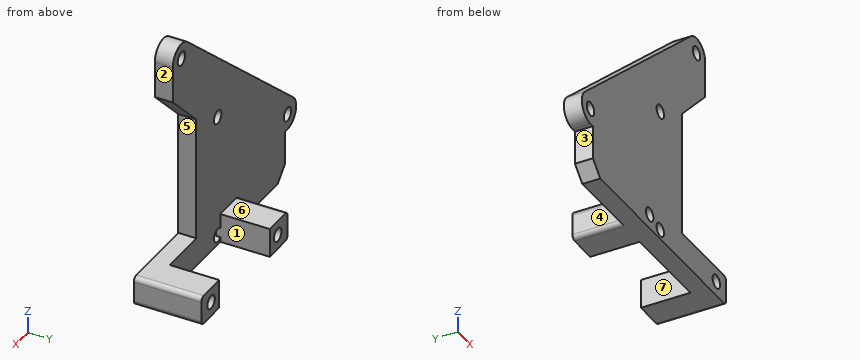
from build123d import *

# Parameters (mm, degrees)
CYLINDER035_R          = 1.5
CYLINDER035_DEPTH      = 30
CYLINDER035_ROLL_ANGLE = -90
CYLINDER034_R          = 1.5
CYLINDER034_DEPTH      = 30
CYLINDER034_ROLL_ANGLE = -90
BOX033_W               = 7.25
BOX033_H               = 12
BOX033_DEPTH           = 6.5
BOX032_W               = 7.25
BOX032_H               = 12
BOX032_DEPTH           = 6.5
SKETCH019_R            = 1.5
PAD017_DEPTH           = 4
FILLET027_R            = 1
CHAMFER008_SIZE        = 3


with BuildPart() as cylinder035:
    # Cylinder035 → Cylinder035 (new body)
    with BuildSketch(Plane.XY):
        Circle(CYLINDER035_R)
    extrude(amount=CYLINDER035_DEPTH)


with BuildPart() as cylinder035_1:
    # Cylinder035 roll: moved
    add(cylinder035.part.rotate(Axis((0, 0, 0), (1, 0, 0)), CYLINDER035_ROLL_ANGLE))


with BuildPart() as cylinder035_2:
    # Cylinder035 placement: moved
    add(cylinder035_1.part.moved(Location((-25, 27, -34.75))))


with BuildPart() as fusion031:
    # Cylinder034 → Cylinder034 (new body)
    with BuildSketch(Plane.XY):
        Circle(CYLINDER034_R)
    extrude(amount=CYLINDER034_DEPTH)


with BuildPart() as fusion031_1:
    # Cylinder034 roll: moved
    add(fusion031.part.rotate(Axis((0, 0, 0), (1, 0, 0)), CYLINDER034_ROLL_ANGLE))


with BuildPart() as fusion031_2:
    # Cylinder034 placement: moved
    add(fusion031_1.part.moved(Location((2, 27, -34.75))))

    # Fusion031: union Cylinder035
    add(cylinder035_2.part)


with BuildPart() as cube033:
    # Box033 → Box033 (new body)
    with BuildSketch(Plane(origin=(-29, 33, -38), x_dir=(1, 0, 0), z_dir=(0, 0, 1))):
        with Locations((3.625, 6)):
            Rectangle(BOX033_W, BOX033_H)
    extrude(amount=BOX033_DEPTH)


with BuildPart() as cube032:
    # Box032 → Box032 (new body)
    with BuildSketch(Plane(origin=(-1.25, 33, -38), x_dir=(1, 0, 0), z_dir=(0, 0, 1))):
        with Locations((3.625, 6)):
            Rectangle(BOX032_W, BOX032_H)
    extrude(amount=BOX032_DEPTH)


with BuildPart() as chamfer008:
    # Sketch019 → Pad017 (new body)
    with BuildSketch(Plane(origin=(0, 30, 0), x_dir=(-1, 0, 0), z_dir=(0, 1, 0))):
        with BuildLine():
            ThreePointArc((8.31768, 16.622663), (4.561577, 17.190758), (2.5, 13.999999))
            Line((2.5, 5.8), (2.5, 13.999999))
            Line((12, -3.7), (2.5, 5.8))
            Line((12, -3.7), (12, -31.5))
            Line((12, -31.5), (-6, -31.5))
            Line((-6, -31.5), (-6, -38))
            Line((48, -38), (-6, -38))
            Line((48, -27.5), (48, -38))
            Line((48, -27.5), (48.999996, -27.5))
            ThreePointArc((48.999996, -27.5), (52.273323, -25.239096), (51.317689, -21.377346))
            Line((8.31768, 16.622663), (51.317689, -21.377346))
        make_face()
        with Locations((6, 14)):
            Circle(SKETCH019_R, mode=Mode.SUBTRACT)
        with Locations((49, -24)):
            Circle(SKETCH019_R, mode=Mode.SUBTRACT)
        with Locations((20.7, -35.85)):
            Circle(SKETCH019_R, mode=Mode.SUBTRACT)
        with Locations((20.7, -8.2)):
            Circle(SKETCH019_R, mode=Mode.SUBTRACT)
    extrude(amount=PAD017_DEPTH)

    # Fusion030: union Cube033, Cube032
    add(cube033.part)
    add(cube032.part)

    # Fillet027
    fillet027_edges = [chamfer008.edges().sort_by_distance(p)[0] for p in [
        (-29, 39.5, -31.5),
        (-29, 39.5, -38),
        (6, 37.5, -38),
        (6, 37.5, -31.5),
    ]]
    fillet(fillet027_edges, radius=FILLET027_R)

    # Cut038: cut Fusion031
    add(fusion031_2.part, mode=Mode.SUBTRACT)

    # Chamfer008
    chamfer008_edges = [chamfer008.edges().sort_by_distance(p)[0] for p in [
        (-48, 32, -38),
    ]]
    chamfer(chamfer008_edges, length=CHAMFER008_SIZE)


solid = chamfer008.part
Input: part model. Units: mm. Frame: model coordinates. Face numbers are marked on the shaded views. A direction names the side the tool comes from. Give positions to 0.01 mm unless a question says otherwise; leave off trailing zeros. Order: outer loops, then holes, each group sorted by start corner. A loop starts at its lowest first (then second) coordinate and runs counter-clockwise, first axis right, second up. Notation, with made-up numbers: (64.25, -38.5) - (113.25, -38.5) arc R24 cw to (113.25, -4.5) - close; hole circle Ø10 at (-32.75, -21). An arc over 180 degrees is marked (long way). Answer as a JSON object with one key per item and string values. Group by question number.
Q1. Line query: probe 1 along Z at (x, y) = (-20.7, 31.5); probe 2 along X at (y, z) = (31.95, -35.85); probe 3 along Z at (x, y) = (-25, 36.75). Output: solid intervals per line, ascending.
Q2. Cut plane A-A, the plane y = 37.5. Output: boundary loops of the cut face in (x, z), then the cut area to 3 significant figures.
Q3. Cut plane C-C, the plane x = -20.7. Output: boundary loops of the cut face in (y, z).
Q4. Mould query, pull axis X, two halves, no side actions, for the marked faces 1, 2 and 3. Classes: pulls with the +X half, pulls with the -X half, needs draft (parallel to the pull), parting line crosses it, or undercut.
Q5. First-contact query: pin 1 Ø7 at (y, z) = (39.5, -36.5) entering from -X; pin 2 Ø1.9 at (x, y) = (-23.5, 38.5) entering from +Z; pin 3 Ø2 at (y, z) = (32.5, 8.5) entering from +X. Flat tips, straight axial feed; report the tip coordinate or a pass-through.
Q6. Set-up query: the marked faces 4, 5, 6 and 7. Return all of +Z, -Z, +X, -X, +Y, -Y with unobstructed straight access to the full face (end or side cutting, diameter ignored); none if empty.
Q7. Cut plane B-B, the plane x = 2. Output: boundary loops of the cut face in (y, z), then the cut area to 3 significant figures.
Q8. Cut plane D-D, the plane z = 11. Output: boundary loops of the cut face in (x, y).
Results:
{
 "1": {"probe 1": "-38 to -37.35, -34.35 to -9.7, -6.7 to 5.68", "probe 2": "-47.15 to -26.02, -23.98 to -22.2, -19.2 to 0.98, 3.02 to 6", "probe 3": "-38 to -36.25, -33.25 to -31.5"},
 "2": {"outline": "(-29, -37) arc R1 ccw to (-28, -38) - (-21.75, -38) - (-21.75, -31.5) - (-28, -31.5) arc R1 ccw to (-29, -32.5) - close; (-1.25, -38) - (5, -38) arc R1 ccw to (6, -37) - (6, -32.5) arc R1 ccw to (5, -31.5) - (-1.25, -31.5) - close; hole circle Ø3 at (-25, -34.75); hole circle Ø3 at (2, -34.75)", "area": "79.3 mm^2"},
 "3": {"outline": "(30, -38) - (34, -38) - (34, -37.35) - (30, -37.35) - close; (30, -34.35) - (34, -34.35) - (34, -9.7) - (30, -9.7) - close; (30, -6.7) - (34, -6.7) - (34, 5.68) - (30, 5.68) - close"},
 "4": {"face 1": "undercut", "face 2": "pulls with the +X half", "face 3": "pulls with the -X half"},
 "5": {"pin 1": "x = -29", "pin 2": "z = -31.5", "pin 3": "x = -2.5"},
 "6": {"face 4": "+Z, -Z, -X, +Y", "face 5": "+X, +Y, -Y", "face 6": "+Z, +X, -X, +Y", "face 7": "+Z, -Z, +Y"},
 "7": {"outline": "(30, -38) - (45, -38) - (45, -36.25) - (30, -36.25) - close; (30, -33.25) - (45, -33.25) - (45, -31.5) - (30, -31.5) - close", "area": "52.5 mm^2"},
 "8": {"outline": "(-14.68, 30) - (-2.5, 30) - (-2.5, 34) - (-14.68, 34) - close"}
}
